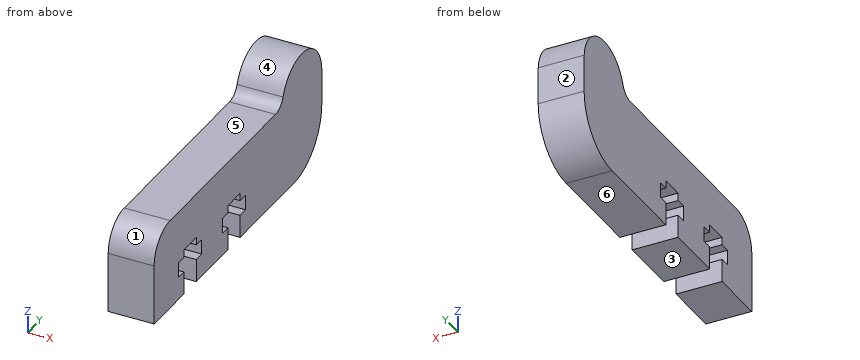
from build123d import *

# Parameters (mm, degrees)
DODANIE_WYCI_GNI_CIE5_DEPTH = 6
WYTNIJ_WYCI_GNI_CIE1_DEPTH  = 20
SZYK_LINIOWY1_COUNT         = 2
SZYK_LINIOWY1_PITCH         = 11


with BuildPart() as part:
    # Szkic8 → Dodanie-wyciągnięcie5 (new body)
    with BuildSketch(Plane(origin=(-151.25, 2.463759923, 0), x_dir=(0, 0, -1), z_dir=(1, 0, 0))):
        with BuildLine():
            Line((0, 53.231732465), (0, 88.231732465))
            ThreePointArc((0, 88.231732465), (-2.050252532, 93.181479934), (-7, 95.231732465))
            Line((-7, 95.231732465), (-11.890119353, 95.231732465))
            Line((-11.890119353, 95.231732465), (-11.889307623, 95.219936285))
            ThreePointArc((-11.889307623, 95.219936285), (-16.499670074, 90.911212793), (-13.219806753, 85.520198357))
            ThreePointArc((-13.219806753, 85.520198357), (-12.255446898, 84.789057353), (-11.889307623, 83.635584713))
            Line((-11.889307623, 83.635584713), (-11.889307623, 57.231732465))
            ThreePointArc((-11.889307623, 57.231732465), (-10.717734748, 54.403305341), (-7.889307623, 53.231732465))
            Line((-7.889307623, 53.231732465), (0, 53.231732465))
        make_face()
    extrude(amount=DODANIE_WYCI_GNI_CIE5_DEPTH)

    # Szkic2 → Wytnij-wyciągnięcie1 (cut)
    with BuildSketch(Plane(origin=(-151.25, 155.607400163, 0), x_dir=(0, 0, -1), z_dir=(-1, 0, 0))):
        Polygon((-6, 81.461907774), (-6, 78.361907774), (-5, 78.361907774), (-5, 76.986907774), (-3, 76.986907774), (-3, 78.361907774), (0, 78.361907774), (0, 81.461907774), (-3, 81.461907774), (-3, 82.836907774), (-5, 82.836907774), (-5, 81.461907774), align=None)
    wytnij_wyci_gni_cie1 = extrude(amount=-WYTNIJ_WYCI_GNI_CIE1_DEPTH, mode=Mode.SUBTRACT)

    # Szyk liniowy1: Wytnij-wyciągnięcie1 ×2
    with Locations(*[(0, -i * SZYK_LINIOWY1_PITCH, 0) for i in range(1, SZYK_LINIOWY1_COUNT)]):
        add(wytnij_wyci_gni_cie1, mode=Mode.SUBTRACT)


solid = part.part
The model under review builds one solid part; all positions refer to its coordinate system, in mm. Face numbers are marked on the shaded views. A direction names the side the tool comes from. Give positions to 0.01 mm unless a question says otherwise; leave off trailing zeros. Order: outer loops, then holes, each group sorted by start corner. A loop starts at its lowest first (then second) coordinate and runs counter-clockwise, first axis right, second up. Notation, with made-up numbers: M -4.5,79.25 L 49.5,79.25 A13 ccw 49.5,88.25 Z; hole C 58,78.25 d4. An arc over 180 degrees is marked long. Use one line per item in the form item = value. Start each with the question number.
Item 1: To check wall thickness, follow line 1 along Z through (x, y) = (-145.55, 62.5); line 2 along Y through (x, z) = (-147.4, 2); line 3 along Z through (x, y) = (-146.85, 80.5). State the ranges of each line that lie inside material, in increasing order. Write a range as from..to.
Item 2: For the marked faces 5 and 6, list the 3-axis set-ups (+Z, -Z, +X, -X, +Y, -Y) from which the entire face can be reached by the end or side of a thin tool; tool diameter is ignored.
Item 3: We need section A-A on z = 3.5. Give the boundary of the cut face in (x, y), plus the area to 3 significant figures.
Item 4: We need section D-D on z = 5.5. Give the boundary of the cut face in (x, y).
Item 5: We need section C-C on y = 69.5. Give the boundary of the cut face in (x, z), plus the area to 3 significant figures.
Item 6: The part is to be moulded in two halves that separate along Y. For the marked faces 1, 2, 3 and 4, say which applies: pulls with the +Y half, pulls with the -Y half, needs draft (parallel to the pull), parting line crosses it, or undercut.
Item 7: Insertion check: pin 1 Ø1.1 at (x, y) = (-149.5, 67) entering from +Z; pin 2 Ø0.9 at (x, y) = (-147.5, 75) entering from -Z; pin 3 Ø2 at (x, z) = (-148.5, 3.5) entering from +Y; pin 4 Ø1 at (x, y) = (-147, 71.5) entering from -Z. Each pin has a flat end and moves straight along its axis. Give the tip position at first contact, or say it passes through.
Completed:
q1.line_1 = 0..3, 5..11.89
q1.line_2 = 55.7..63.15, 66.25..74.15, 77.25..95.59
q1.line_3 = 0..11.89
q2.face_5 = +Z, +X, -X, -Y
q2.face_6 = -Z, +X, -X, +Y, -Y
q3.outline = M -151.25,55.7 L -145.25,55.7 L -145.25,61.77 L -151.25,61.77 Z; M -151.25,67.62 L -145.25,67.62 L -145.25,72.77 L -151.25,72.77 Z; M -151.25,78.62 L -145.25,78.62 L -145.25,96.76 L -151.25,96.76 Z
q3.area = 176 mm²
q4.outline = M -151.25,55.7 L -145.25,55.7 L -145.25,63.15 L -151.25,63.15 Z; M -151.25,66.25 L -145.25,66.25 L -145.25,74.15 L -151.25,74.15 Z; M -151.25,77.25 L -145.25,77.25 L -145.25,97.53 L -151.25,97.53 Z
q5.outline = M -151.25,0 L -145.25,0 L -145.25,11.89 L -151.25,11.89 Z
q5.area = 71.3 mm²
q6.face_1 = pulls with the -Y half
q6.face_2 = pulls with the +Y half
q6.face_3 = needs draft
q6.face_4 = parting line crosses it
q7.pin_1 = 11.89
q7.pin_2 = 6
q7.pin_3 = 97.23
q7.pin_4 = 0
